```python
from build123d import *

# Parameters (mm, degrees)
SKETCH1_W           = 139.7
SKETCH1_H           = 12.7
BOSS_EXTRUDE1_DEPTH = 5.08
SKETCH3_W           = 25.4
SKETCH3_H           = 2.54
CUT_EXTRUDE1_DEPTH  = 17.78
SKETCH4_R           = 1.0795
CUT_EXTRUDE2_DEPTH  = 17.78


with BuildPart() as part:
    # Sketch1 → Boss-Extrude1 (new body)
    with BuildSketch(Plane(origin=(0, 0, 0), x_dir=(1, 0, 0), z_dir=(0, 1, 0))):
        Rectangle(SKETCH1_W, SKETCH1_H)
    extrude(amount=BOSS_EXTRUDE1_DEPTH)

    # Sketch3 → Cut-Extrude1 (cut)
    with BuildSketch(Plane.XY.offset(6.35)):
        with Locations((57.15, 3.81)):
            Rectangle(SKETCH3_W, SKETCH3_H)
    extrude(amount=-CUT_EXTRUDE1_DEPTH, mode=Mode.SUBTRACT)

    # Sketch4 → Cut-Extrude2 (cut)
    with BuildSketch(Plane(origin=(0, 2.54, 0), x_dir=(1, 0, 0), z_dir=(0, 1, 0))):
        with Locations((57.15, 0)):
            Circle(SKETCH4_R)
    extrude(amount=-CUT_EXTRUDE2_DEPTH, mode=Mode.SUBTRACT)


solid = part.part
```
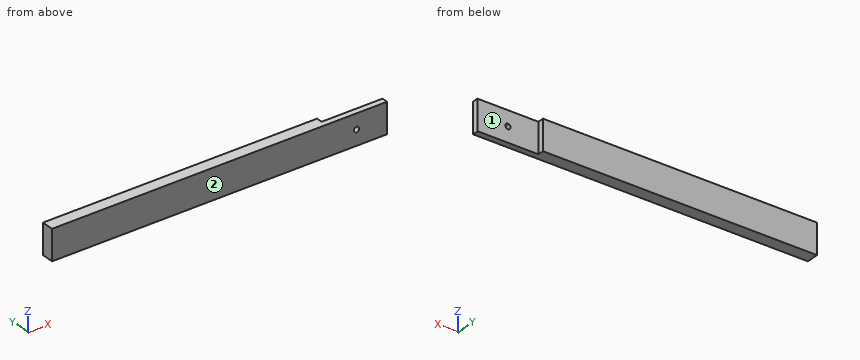
Input: part model. Units: mm. Frame: model coordinates. Face numbers are marked on the shaded views. A direction names the side the tool comes from. Give positions to 0.01 mm unless a question says otherwise; leave off trailing zeros. Loops run counter-clockwise (first coordinate to the right, second up) from the corner with the lowest first, then second, coordinate; pieces in that order, holes last.
1) Section query A-A on y = 4.2. Return the cut outline in (x, z).
A:
outline: (-69.85, -6.35) - (44.45, -6.35) - (44.45, 6.35) - (-69.85, 6.35) - close
2) Reachability of the marked faces 1 and 2 from +Z, -Z, +X, -X, +Y, -Y: full face, straight path, thin tool, end or side. Return the list, or none.
A:
face 1: +Z, -Z, +X, +Y
face 2: +Z, -Z, +X, -X, -Y
3) Line query: L1, parallel to Z at x = 57.15, y = 1.8; L2, parallel to X at y = 2.05, z = 0; L3, parallel to X at y = 4.7, z = 5. Output: solid intervals per line, ascending.
A:
L1: z = -6.35 to -1.08, 1.08 to 6.35
L2: x = -69.85 to 56.07, 58.23 to 69.85
L3: x = -69.85 to 44.45
4) Section query B-B on x = 49.5. Return the cut outline in (y, z), and give its area (3 significant figures).
A:
outline: (0, -6.35) - (2.54, -6.35) - (2.54, 6.35) - (0, 6.35) - close
area: 32.3 mm2
5) Contact query for a flat-ended pin moving along its axis: pin 1 (1.5 mm diameter, centred on y = 3.5, z = 2, fed in from +X). Output: stop coordinate, or through.
A:
pin 1: stops at x = 44.45
